Part model, mm, in its own coordinate system. A direction names the side the tool comes from. Give positions to 0.01 mm unless a question says otherwise; leave off trailing zeros. Write each loop counter-clockwise with the first axis right and the second up, starting at its lowest first coordinate (ties: lowest second). Pieces come first, ordered by that corner, then holes. Notation, with made-up numbers: M 23.25,21.5 L 71.25,21.5 A20 ccw 71.25,36.5 Z; hole C 85,-35.75 d1. An arc over 180 degrees is marked long. Use CSV: the item, a comma, the result in double quotes. Start each with the question number.
1. Band-saw the part on B-B, the plane y = 0. List the corners of the cut face in (x, z), then the cut area to 3 significant figures.
2. Band-saw the part on A-A, the plane z = 2.6. List the corners of the cut face in (x, y), then the cut area to 3 significant figures.
3. 3-axis set-ups, long thin cutter, end or side, ignore diameter. For faces 1 (the face through (-7, 0, 3)), 2 (the face through (-5.5, 0, 2)): which of +Z, -Z, +X, -X, +Y, -Y reach the whole face in a straight line?
4. Drill centre lines: line 1 along X through (y, z) = (0, 1.5); line 2 along Z through (x, y) = (1.75, -4.5). Where is each one in solid material? Low to high. Write a range as from..to.
5. Band-saw the part on C-C, the plane x = -5.25. List the corners of the cut face in (y, z), then the cut area to 3 significant figures.
6. Drop a flat-ended pin along its axis: pin 1 Ø1 at (x, y) = (-4.5, -3) entering from +Z. Give the stop position or say it passes through.
from build123d import *

# Parameters (mm, degrees)
F0_W     = 3
F0_H     = 11
F1_DEPTH = 3
F0_W_2   = 11
F2_DEPTH = 1
F3_R     = 0.5


with BuildPart() as f1:
    # F0 (on Top) → F1 (new body)
    with BuildSketch(Plane.XY):
        with Locations((-7, 0)):
            Rectangle(F0_W, F0_H)
        with Locations((7, 0)):
            Rectangle(F0_W, F0_H)
    extrude(amount=F1_DEPTH)

    # F0 (on Top) → F2 (join)
    with BuildSketch(Plane.XY):
        Rectangle(F0_W_2, F0_H)
    extrude(amount=F2_DEPTH)

    # F3
    f3_edges = [f1.edges().sort_by_distance(p)[0] for p in [
        (-5.5, -5.5, 2),
        (5.5, -5.5, 2),
        (8.5, -5.5, 1.5),
        (8.5, 5.5, 1.5),
        (-8.5, -5.5, 1.5),
        (-5.5, 5.5, 2),
        (-8.5, 5.5, 1.5),
        (5.5, 5.5, 2),
    ]]
    fillet(f3_edges, radius=F3_R)


solid = f1.part
Output:
1,outline,"M -8.5,0 L 8.5,0 L 8.5,3 L 5.5,3 L 5.5,1 L -5.5,1 L -5.5,3 L -8.5,3 Z"
1,area,"29.0 mm²"
2,outline,"M -8.5,-5 A0.5 ccw -8,-5.5 L -6,-5.5 A0.5 ccw -5.5,-5 L -5.5,5 A0.5 ccw -6,5.5 L -8,5.5 A0.5 ccw -8.5,5 Z; M 5.5,-5 A0.5 ccw 6,-5.5 L 8,-5.5 A0.5 ccw 8.5,-5 L 8.5,5 A0.5 ccw 8,5.5 L 6,5.5 A0.5 ccw 5.5,5 Z"
2,area,"65.6 mm²"
3,face 1,"+Z, +X, -X, +Y, -Y"
3,face 2,"+Z, +Y, -Y"
4,line 1,"x = -8.5..-5.5, 5.5..8.5"
4,line 2,"z = 0..1"
5,outline,"M -5.5,0 L 5.5,0 L 5.5,1 L -5.5,1 Z"
5,area,"11.0 mm²"
6,pin 1,"stops at z = 1"
